Here's how the part is built. I have some questions about the finished solid (model axes, mm). Round coordinates to 2 decimals unless told otherwise and drop trailing zeros. Write each loop counter-clockwise with the first axis right and the second up, starting at its lowest first coordinate (ties: lowest second). Pieces come first, ordered by that corner, then holes. Notation, with made-up numbers: M 56.25,-30.5 L 109.25,-30.5 A33 cw 109.25,-1.5 Z; hole C 80.5,22.25 d7. An arc over 180 degrees is marked long. Use a Markdown table: item, result. Add a question column.
Autodesk Inventor part; units mm, degrees
ref_plane "YZ Plane" through (0, 0, 0) normal (1, 0, 0) x (0, 1, 0)
ref_plane "XZ Plane" through (0, 0, 0) normal (0, 1, 0) x (-1, 0, 0)
ref_plane "XY Plane" through (0, 0, 0) normal (0, 0, 1) x (1, 0, 0)
sketch "Sketch1" plane through (0, 0, 0) normal (0, 0, 1) x (1, 0, 0)
  line L0 (-1.3279, 2.3) -> (1.3279, 2.3)
  line L1 (0, 2.3) -> (0, 0) construction
  circle A0 centre (0, 0) radius 2.3 construction
  line L2 (-2.656, 0) -> (-1.3279, 2.3)
  line L3 (-1.9919, 1.15) -> (0, 0) construction
  line L4 (-1.3282, -2.3001) -> (-2.656, 0)
  line L5 (-1.9919, -1.15) -> (0, 0) construction
  line L6 (1.3277, -2.3001) -> (-1.3282, -2.3001)
  line L7 (0, -2.3) -> (0, 0) construction
  line L8 (2.6557, -0.0001) -> (1.3277, -2.3001)
  line L9 (1.9919, -1.15) -> (0, 0) construction
  line L10 (1.3279, 2.3) -> (2.6557, -0.0001)
  line L11 (1.9919, 1.15) -> (0, 0) construction
  circle A1 centre (0, 0) radius 1.375
  point P0 (-2.656, 0)
  point P1 (2.6557, -0.0001)
  point P2 (-2.656, 0)
  dimension "d8" = 120
  dimension "d9" = 120.003
  dimension "d11" = 4.6
  dimension "d0" = 2.3
  dimension "d13" = 2.75
extrude "Extrusion1" add sketch "Sketch1" along normal blind 16
properties part number "spacer"
Item 1: For pin 1 Ø1.6 at (x, y) = (0, 0) entering from +Z, with a flat end and sliding along its axis, tell me the tip position at first contact or that it passes through.
Item 2: If we mould it in two halves opening along Y, with no side actions, what happens to faces 1 (the face through (-0.3, 1.34, 7.89)), 2 (the face through (-1.98, -1.17, 7.89)), 3 (the face through (0, 2.3, 8)), 4 (the face through (1.1, 1.1, 0))? For each: +Y half, -Y half, draft (parallel to the pull), parting line (faces both ways), or undercut.
Item 3: Imagine slicing it at B-B on z = 6.5. List the corners of the cut face in (x, y) for me (3 decimals), plus the area to 3 significant figures.
Item 4: Imagine slicing it at C-C on y = -0.6. List the corners of the cut face in (x, z) for me.
Item 5: Imagine slicing it at A-A on x = 0. List the corners of the cut face in (y, z) for me (3 decimals).
Item 6: I need wall thicknesses on probe 1 along Y at (x, z) = (-0.1, 6.5); probe 2 along Y at (x, z) = (-0.5, 10.25); probe 3 along X at (y, z) = (0.3, 7.25). Which ranges of each line are inside material? Lowest first, please. Write a range as from..to.
Item 7: Imagine slicing it at D-D on x = 1.75. List the corners of the cut face in (y, z) for me.
The answers:
| question | item | result |
|---|---|---|
| 1 | pin 1 | through |
| 2 | face 1 | undercut |
| 2 | face 2 | -Y half |
| 2 | face 3 | +Y half |
| 2 | face 4 | draft |
| 3 | outline | M -2.656,0 L -1.328,-2.3 L 1.328,-2.3 L 2.656,0 L 1.328,2.3 L -1.328,2.3 Z; hole C 0,0 d2.75 |
| 3 | area | 12.4 mm² |
| 4 | outline | M -2.31,0 L -1.24,0 L -1.24,16 L -2.31,16 Z; M 1.24,0 L 2.31,0 L 2.31,16 L 1.24,16 Z |
| 5 | outline | M -2.3,0 L -1.375,0 L -1.375,16 L -2.3,16 Z; M 1.375,0 L 2.3,0 L 2.3,16 L 1.375,16 Z |
| 6 | probe 1 | -2.3..-1.37, 1.37..2.3 |
| 6 | probe 2 | -2.3..-1.28, 1.28..2.3 |
| 6 | probe 3 | -2.48..-1.34, 1.34..2.48 |
| 7 | outline | M -1.57,0 L 1.57,0 L 1.57,16 L -1.57,16 Z |
